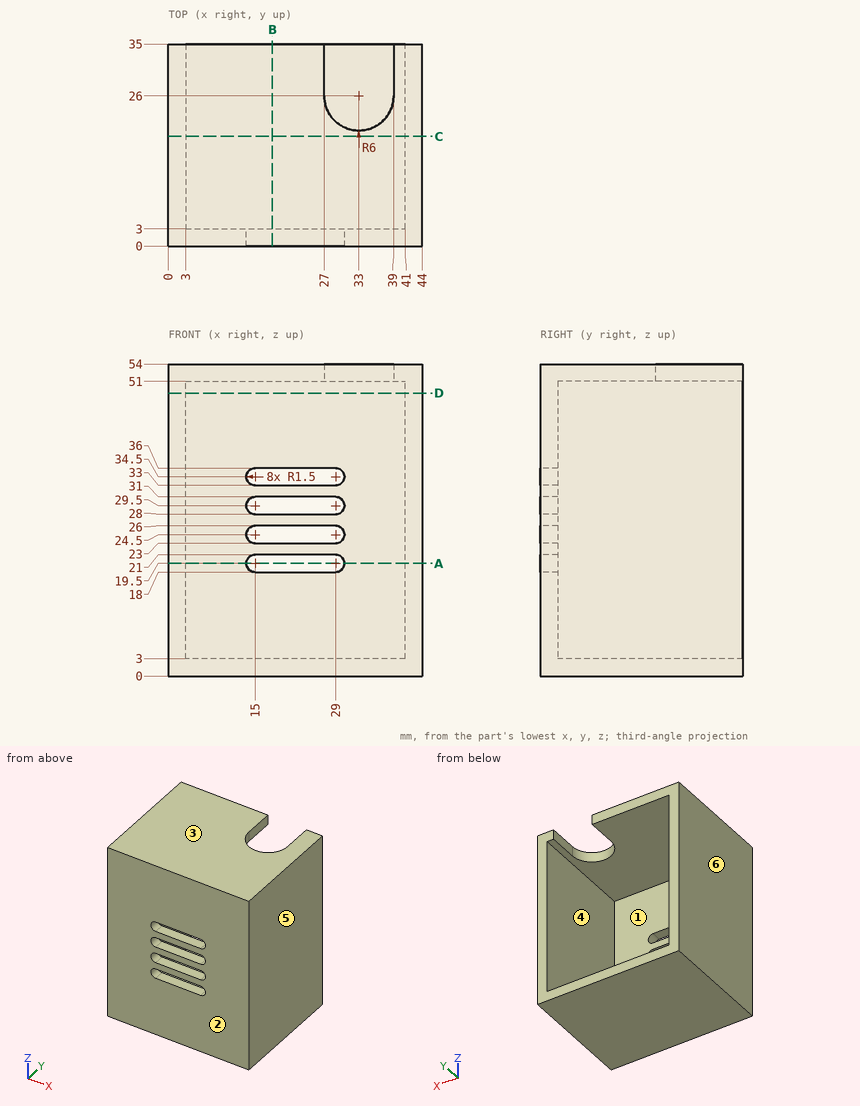
Geometry check sheet. Reference: drawing and pictorial views, mm from the part's lowest x, y, z. A direction names the side the tool comes from. Round coordinates to 2 decimals unless told otherwise and drop trailing zeros. Write each loop counter-clockwise with the first axis right and the second up, starting at its lowest first coordinate (ties: lowest second). Pieces come first, ordered by that corner, then holes. Notation, with made-up numbers: (-6, 50) -> (52, 50) arc R9 ccw to (52, 61) -> close; hole circle Ø5 at (51.5, -4.75). An arc over 180 degrees is marked (long way). Put each result on its own line as item: value.
1) Cross-section at C-C, the plane y = 19. Enter the section's corners in (x, z).
Recorded:
outline: (0, 0) -> (44, 0) -> (44, 54) -> (0, 54) -> close; hole (3, 3) -> (41, 3) -> (41, 51) -> (3, 51) -> close
2) Cross-section at A-A, the plane z = 19.5. Enter the section's corners in (x, y).
Recorded:
outline: (0, 0) -> (13.5, 0) -> (13.5, 3) -> (3, 3) -> (3, 35) -> (0, 35) -> close; (30.5, 0) -> (44, 0) -> (44, 35) -> (41, 35) -> (41, 3) -> (30.5, 3) -> close
3) Access from +Z, -Z, +X, -X, +Y, -Y to the whole of each face (thin tool, end or side, straight path). Record for the marked faces 1 and 2.
Recorded:
face 1: +Y
face 2: +Z, -Z, +X, -X, -Y
4) Depth check by flat-ended pin: P1, Ø6, axis at x = 27, z = 22, coming from the +Y side; P2, Ø6, axis at x = 31, y = 26.5, coming from the +Z side. Enter the tip coordinate at first touch or a pass-through.
Recorded:
P1: stops at y = 3
P2: stops at z = 3
5) Thickness scan on probe 1 along Z at (x, y) = (17, 6.5); probe 2 along X at (y, z) = (24, 39.5); probe 3 along Y at (x, z) = (30, 22). Record the ranges inside material, lowest first. Write a range as from..to.
Recorded:
probe 1: z = 0..3, 51..54
probe 2: x = 0..3, 41..44
probe 3: y = 0..3
6) Cross-section at D-D, the plane z = 49. Enter the section's corners in (x, y), plus the area to 3 significant figures.
Recorded:
outline: (0, 0) -> (44, 0) -> (44, 35) -> (41, 35) -> (41, 3) -> (3, 3) -> (3, 35) -> (0, 35) -> close
area: 324 mm2
7) Cross-section at B-B, the plane x = 18. Enter the section's corners in (y, z), plus the area to 3 significant figures.
Recorded:
outline: (0, 0) -> (35, 0) -> (35, 3) -> (3, 3) -> (3, 18) -> (0, 18) -> close; (0, 21) -> (3, 21) -> (3, 23) -> (0, 23) -> close; (0, 26) -> (3, 26) -> (3, 28) -> (0, 28) -> close; (0, 31) -> (3, 31) -> (3, 33) -> (0, 33) -> close; (0, 36) -> (3, 36) -> (3, 51) -> (35, 51) -> (35, 54) -> (0, 54) -> close
area: 318 mm2
8) Release check for a two-part mould opening along X. For the marked faces 3, 4, 5 and 6 record: pulls with the +X half, pulls with the -X half, needs draft (parallel to the pull), parting line crosses it, or undercut.
Recorded:
face 3: needs draft
face 4: undercut
face 5: pulls with the +X half
face 6: pulls with the -X half
